Check sheet for the modelled part. Datum: model origin and axes. Units: mm. Round coordinates to 2 decimals unless told otherwise and drop trailing zeros. Order: outer loops, then holes, each group sorted by start corner. A loop starts at its lowest first (then second) coordinate and runs counter-clockwise, first axis right, second up. Notation, with made-up numbers: (8.5, -33) -> (12.5, -33) arc R15 cw to (12.5, -6) -> close; hole circle Ø5 at (49.25, 55.25). An arc over 180 degrees is marked (long way). Use CSV: the item, a comma, the result in double quotes.
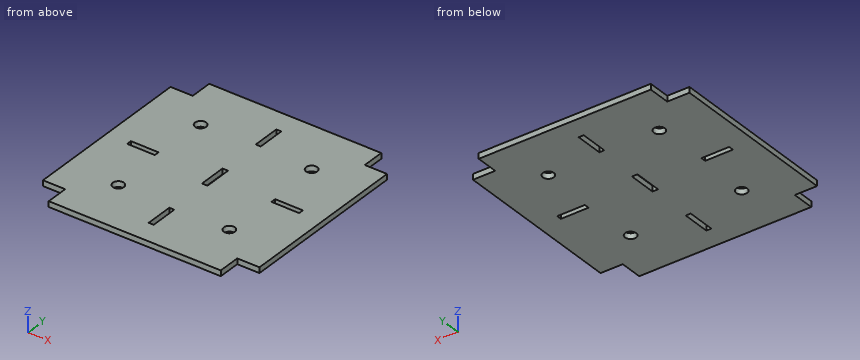
```python
from build123d import *

# Parameters (mm, degrees)
SKETCH_1_R      = 2
SKETCH_1_W      = 1.8
SKETCH_1_H      = 10
SKETCH_1_W_2    = 10
SKETCH_1_H_2    = 1.8
SKETCH_1_W_3    = 2
EXTRUDE_1_DEPTH = 2


with BuildPart() as part:
    # 草圖1 → 填料-伸長1 (new body)
    with BuildSketch(Plane.XY):
        Polygon((-31, 39), (31, 39), (31, 31), (39, 31), (39, -31), (31, -31), (31, -39), (-31, -39), (-31, -31), (-39, -31), (-39, 31), (-31, 31), align=None)
        with Locations((-20, 20)):
            Circle(SKETCH_1_R, mode=Mode.SUBTRACT)
        with Locations((20, 20)):
            Circle(SKETCH_1_R, mode=Mode.SUBTRACT)
        with Locations((20, -20)):
            Circle(SKETCH_1_R, mode=Mode.SUBTRACT)
        with Locations((-20, -20)):
            Circle(SKETCH_1_R, mode=Mode.SUBTRACT)
        with Locations((0, -26)):
            Rectangle(SKETCH_1_W, SKETCH_1_H, mode=Mode.SUBTRACT)
        with Locations((0, 26)):
            Rectangle(SKETCH_1_W, SKETCH_1_H, mode=Mode.SUBTRACT)
        with Locations((-26, 0)):
            Rectangle(SKETCH_1_W_2, SKETCH_1_H_2, mode=Mode.SUBTRACT)
        with Locations((26, 0)):
            Rectangle(SKETCH_1_W_2, SKETCH_1_H_2, mode=Mode.SUBTRACT)
        Rectangle(SKETCH_1_W_3, SKETCH_1_H, mode=Mode.SUBTRACT)
    extrude(amount=EXTRUDE_1_DEPTH)


solid = part.part
```
Q1. Go/stop test with flat-tipped pins: pin 1 (0.6 mm diameter, centred on y = 35, z = 1.5, fed in from -X); pin 2 (0.6 mm diameter, centred on x = -36, z = 1, fed in from +Y). Record where each tip stops, or that it passes through.
Result sheet:
pin 1,"stops at x = -31"
pin 2,"stops at y = 31"
Q2. Sectioned sample at B-B, the plane x = -20. Enter the section's corners in (y, z).
Result sheet:
outline,"(-39, 0) -> (-22, 0) -> (-22, 2) -> (-39, 2) -> close; (-18, 0) -> (18, 0) -> (18, 2) -> (-18, 2) -> close; (22, 0) -> (39, 0) -> (39, 2) -> (22, 2) -> close"
Q3. Sectioned sample at A-A, the plane y = -26.5. Enter the section's corners in (x, z).
Result sheet:
outline,"(-39, 0) -> (-0.9, 0) -> (-0.9, 2) -> (-39, 2) -> close; (0.9, 0) -> (39, 0) -> (39, 2) -> (0.9, 2) -> close"
Q4. Scan lines: L1, parallel to Y at x = -20, z = 0.95; L2, parallel to X at y = 4.5, z = 1.6; L3, parallel to X at y = 28.5, z = 0.45. Record each from-to range of solid material in increasing order.
Result sheet:
L1,"y = -39 to -22, -18 to 18, 22 to 39"
L2,"x = -39 to -1, 1 to 39"
L3,"x = -39 to -0.9, 0.9 to 39"
